from build123d import *

# Parameters (mm, degrees)
ESQUISSE1_W             = 104.6
ESQUISSE1_H             = 90
BOSS_EXTRU_3_DEPTH      = 6
ENL_V_MAT_EXTRU_1_DEPTH = 91
ENL_V_MAT_EXTRU_2_DEPTH = 91
ENL_V_MAT_EXTRU_4_DEPTH = 90


with BuildPart() as part:
    # Esquisse1 → Boss.-Extru.3 (new body)
    with BuildSketch(Plane.XY):
        with Locations((-0.339287382, -16.126157407)):
            Rectangle(ESQUISSE1_W, ESQUISSE1_H)
    extrude(amount=BOSS_EXTRU_3_DEPTH)

    # Esquisse4 → Enlèv. mat.-Extru.1 (cut)
    with BuildSketch(Plane.XZ.offset(61.126157407)):
        Polygon((-49.138987395, 6), (-52.639287382, 6), (-52.639287382, 3), align=None)
    extrude(amount=-ENL_V_MAT_EXTRU_1_DEPTH, mode=Mode.SUBTRACT)

    # Esquisse5 → Enlèv. mat.-Extru.2 (cut)
    with BuildSketch(Plane.XZ.offset(61.126157407)):
        Polygon((-52.639287382, 3), (-49.139287382, 0), (-52.639287382, 0), align=None)
    extrude(amount=-ENL_V_MAT_EXTRU_2_DEPTH, mode=Mode.SUBTRACT)

    # Esquisse7 → Enlèv. mat.-Extru.4 (cut)
    with BuildSketch(Plane(origin=(0, -61.126157407, 0), x_dir=(-1, 0, 0), z_dir=(0, -1, 0))):
        Polygon((49.138987395, -6), (50.889137389, -4.5), (49.138987395, -4.6198399), align=None)
    extrude(amount=-ENL_V_MAT_EXTRU_4_DEPTH, mode=Mode.SUBTRACT)


solid = part.part
Work out the finished part from the listing and answer in its coordinate system (mm). Round coordinates to 2 decimals unless told otherwise and drop trailing zeros. Write each loop counter-clockwise with the first axis right and the second up, starting at its lowest first coordinate (ties: lowest second). Pieces come first, ordered by that corner, then holes.
1) A cutting plane is placed at A-A (y = -50). Give the vertices of the cut face in (x, z), plus the area to 3 significant figures.
2) A cutting plane is placed at B-B (z = 1.1). Give the vertices of the cut face in (x, y), plus the area to 3 significant figures.
3) Given pin 1 Ø1.5 at (y, z) = (-30.5, 5.5) entering from -X, flat-ended and moving along its own axis, determine where the tip first touches the part or whether it passes through.
4) Straight lines are drawn through the part: line 1 (X direction, y = -57, z = 5.3); line 2 (X direction, y = -51.5, z = 2.55). For each, find the intervals that lie inside material, in ascending order.
Completed:
1. outline: (-52.64, 3) - (-49.14, 0) - (51.96, 0) - (51.96, 6) - (-49.14, 6) - (-49.14, 4.62) - (-50.89, 4.5) - close
1. area: 616 mm2
2. outline: (-50.42, -61.13) - (51.96, -61.13) - (51.96, 28.87) - (-50.42, 28.87) - close
2. area: 9,210 mm2
3. pin 1: stops at x = -49.14
4. line 1: x = -49.14 to 51.96
4. line 2: x = -52.11 to 51.96
